from build123d import *

# Parameters (mm, degrees)
F0_W      = 86
F0_H      = 61
F0_W_2    = 80
F0_H_2    = 55
F1_DEPTH  = 67
F2_DEPTH  = 6
F3_W      = 80
F3_H      = 5.4
F4_DEPTH  = 3
F6_W      = 28
F6_H      = 3
F6_H_2    = 55
F7_DEPTH  = 35
F8_R      = 13.99999
F9_DEPTH  = 23
F10_W     = 28
F10_H     = 29.4785189629
F11_DEPTH = 25
F12_W     = 6
F12_H     = 2
F13_DEPTH = 6
F14_R     = 1


# Not quite as in the source:
# - a fillet or chamfer is up to 0.001 mm smaller than in the source, because OpenCascade refuses the exact size


with BuildPart() as f1:
    # F0 (on Top) → F1 (new body)
    with BuildSketch(Plane.XY):
        Rectangle(F0_W, F0_H)
        Rectangle(F0_W_2, F0_H_2, mode=Mode.SUBTRACT)
    extrude(amount=F1_DEPTH)

    # F0 (on Top) → F2 (join)
    with BuildSketch(Plane.XY):
        Rectangle(F0_W_2, F0_H_2)
    extrude(amount=F2_DEPTH)

    # F3 (on face) → F4 (cut)
    with BuildSketch(Plane.XZ.offset(30.5)):
        with Locations((0, 8.7)):
            Rectangle(F3_W, F3_H)
    extrude(amount=-F4_DEPTH, mode=Mode.SUBTRACT)

    # F6 (on face) → F7 (cut)
    with BuildSketch(Plane.XY):
        with Locations((0, -29)):
            Rectangle(F6_W, F6_H)
        Rectangle(F6_W, F6_H_2)
        with Locations((0, 29)):
            Rectangle(F6_W, F6_H)
    extrude(amount=F7_DEPTH, mode=Mode.SUBTRACT)

    # F8 (radius 14 in the source; OpenCascade refuses exactly that, so slightly less here)
    f8_edges = [f1.edges().sort_by_distance(p)[0] for p in [
        (14, -29, 35),
        (-14, -29, 35),
        (-14, 29, 35),
        (14, 29, 35),
    ]]
    fillet(f8_edges, radius=F8_R)

    # F5 (on Right) → F9 (join, symmetric)
    with BuildSketch(Plane.YZ):
        Polygon((-10.8611155301, 0), (29.1388844699, 0), (29.1388844699, 12), (-10.8611155301, 6), align=None)
    extrude(amount=F9_DEPTH, both=True)

    # F10 (on face) → F11 (cut)
    with BuildSketch(Plane(origin=(0, -1.1191932513, 7.4612883418), x_dir=(1, 0, 0), z_dir=(0, -0.1483404529, 0.9889363529))):
        Polygon((-14, -9.8509092629), (14, -9.8509092629), (14, 28.9393682094), (14, 30.5965875694), (-14, 30.5965875694), (-14, 28.9393682094), align=None)
        with Locations((0, -24.5901687443)):
            Rectangle(F10_W, F10_H)
    extrude(amount=-F11_DEPTH, mode=Mode.SUBTRACT)

    # F12 (on face) → F13 (cut)
    with BuildSketch(Plane(origin=(0, 30.5, 0), x_dir=(-1, 0, 0), z_dir=(0, 1, 0))):
        with BuildLine():
            Line((-31, 55.5), (-31, 59.5))
            ThreePointArc((-31, 59.5), (-33, 57.5), (-31, 55.5))
        make_face()
        Polygon((-25, 57.5), (-19, 57.5), (-19, 59.5), (-31, 59.5), (-31, 55.5), (-25, 55.5), align=None)
        with Locations((-22, 56.5)):
            Rectangle(F12_W, F12_H)
        with BuildLine():
            ThreePointArc((-19, 55.5), (-17.5857864376, 56.0857864376), (-17, 57.5))
            Line((-17, 57.5), (-19, 57.5))
            Line((-19, 57.5), (-19, 55.5))
        make_face()
        with BuildLine():
            Line((-19, 57.5), (-17, 57.5))
            ThreePointArc((-17, 57.5), (-17.5857864376, 58.9142135624), (-19, 59.5))
            Line((-19, 59.5), (-19, 57.5))
        make_face()
        with BuildLine():
            Line((19, 55.5), (19, 57.5))
            Line((19, 57.5), (17, 57.5))
            ThreePointArc((17, 57.5), (17.5857864376, 56.0857864376), (19, 55.5))
        make_face()
        with BuildLine():
            Line((17, 57.5), (19, 57.5))
            Line((19, 57.5), (19, 59.5))
            ThreePointArc((19, 59.5), (17.5857864376, 58.9142135624), (17, 57.5))
        make_face()
        Polygon((19, 57.5), (25, 57.5), (25, 55.5), (31, 55.5), (31, 59.5), (19, 59.5), align=None)
        with Locations((22, 56.5)):
            Rectangle(F12_W, F12_H)
        with BuildLine():
            Line((31, 59.5), (31, 55.5))
            ThreePointArc((31, 55.5), (33, 57.5), (31, 59.5))
        make_face()
    extrude(amount=-F13_DEPTH, mode=Mode.SUBTRACT)

    # F14
    f14_edges = [f1.edges().sort_by_distance(p)[0] for p in [
        (-43, -30.5, 33.5),
        (43, -30.5, 33.5),
        (43, 30.5, 33.5),
        (-43, 30.5, 33.5),
    ]]
    fillet(f14_edges, radius=F14_R)


solid = f1.part
For this review, take the finished solid that the model builds, in its own axes (mm). A direction names the side the tool comes from. Give positions to 0.01 mm unless a question says otherwise; leave off trailing zeros. Loops run counter-clockwise (first coordinate to the right, second up) from the corner with the lowest first, then second, coordinate; pieces in that order, holes last.
Item 1: Tool access review of faces 1 (the cylindrical face through (-10, -29, 30.8)), 2 (the flat face through (-30, -2, 6)), 3 (the flat face through (25, 29, 59.5)): name each direction out of +Z, -Z, +X, -X, +Y, -Y from which nothing blocks a thin tool from reaching the whole face with its end or side.
Item 2: Take a section at B-B, the plane x = 37.5. State the section outline as (y, z) points, and give its area (3 significant figures).
Item 3: Take a section at C-C, the plane y = 26. State the section outline as (x, z) points, and give its area (3 significant figures).
Item 4: Take a section at D-D, the plane z = 16. State the section outline as (x, y) points.
Item 5: For line 1 along X through (y, z) = (24, 17.5); line 2 along Y through (x, z) = (38.5, 13); line 3 along Z through (x, y) = (-33.5, -22), list the stretches that pass through material, from the lowest coordinate up.
Item 6: Take a section at A-A, the plane z = 53. State the section outline as (x, y) points.
Item 7: Insertion check: pin 1 (2 mm diameter, centred on x = -12.5, y = -21, fed in from +Z); pin 2 (13 mm diameter, centred on x = -33, y = -2, fed in from +Z); pin 3 (5 mm diameter, centred on x = 19, y = 2.5, fed in from +Z). Each pin has a flat end and moves straight along its axis. Give the tip position at first contact, or say it passes through.
Item 8: Draft analysis for pull direction Y (two halves, no side actions). For faces 4 (the flat face through (-25, 29, 59.5)), 5 (the flat face through (-1, -27.5, 39)), state which applies: +Y half, -Y half, draft (parallel to the pull), parting line (faces both ways), or undercut.
Calculated:
1. face 1: -Z, +Y, -Y
1. face 2: -Y
1. face 3: +Y
2. outline: (-30.5, 0) - (30.5, 0) - (30.5, 67) - (27.5, 67) - (27.5, 6) - (-30.5, 6) - close; (-30.5, 11.4) - (-27.5, 11.4) - (-27.5, 67) - (-30.5, 67) - close
2. area: 716 mm2
3. outline: (-43, 0) - (-14, 0) - (-14, 11.53) - (-23, 11.53) - (-23, 6) - (-40, 6) - (-40, 67) - (-43, 67) - close; (14, 0) - (43, 0) - (43, 67) - (40, 67) - (40, 6) - (23, 6) - (23, 11.53) - (14, 11.53) - close
3. area: 814 mm2
4. outline: (-43, -29.5) arc R1 ccw to (-42, -30.5) - (-14, -30.5) - (-14, -27.5) - (-40, -27.5) - (-40, 27.5) - (-14, 27.5) - (-14, 30.5) - (-42, 30.5) arc R1 ccw to (-43, 29.5) - close; (14, -30.5) - (42, -30.5) arc R1 ccw to (43, -29.5) - (43, 29.5) arc R1 ccw to (42, 30.5) - (14, 30.5) - (14, 27.5) - (40, 27.5) - (40, -27.5) - (14, -27.5) - close
5. line 1: x = -43 to -40, 40 to 43
5. line 2: y = -30.5 to -27.5, 27.5 to 30.5
5. line 3: z = 0 to 6
6. outline: (-43, -29.5) arc R1 ccw to (-42, -30.5) - (42, -30.5) arc R1 ccw to (43, -29.5) - (43, 29.5) arc R1 ccw to (42, 30.5) - (-42, 30.5) arc R1 ccw to (-43, 29.5) - close; hole (-40, -27.5) - (40, -27.5) - (40, 27.5) - (-40, 27.5) - close
7. pin 1: passes through
7. pin 2: stops at z = 6
7. pin 3: stops at z = 8.38
8. face 4: draft
8. face 5: undercut
